```python
from build123d import *

# Parameters (mm, degrees)
SKETCH1_W           = 60
SKETCH1_H           = 50
BOSS_EXTRUDE1_DEPTH = 30
CUT_EXTRUDE1_DEPTH  = 30
BOSS_EXTRUDE2_DEPTH = 20
BOSS_EXTRUDE3_DEPTH = 30


with BuildPart() as part:
    # Sketch1 → Boss-Extrude1 (new body)
    with BuildSketch(Plane(origin=(0, 0, 0), x_dir=(1, 0, 0), z_dir=(0, 1, 0))):
        with Locations((30, 25)):
            Rectangle(SKETCH1_W, SKETCH1_H)
    extrude(amount=BOSS_EXTRUDE1_DEPTH)

    # Sketch2 → Cut-Extrude1 (cut)
    with BuildSketch(Plane(origin=(0, 30, 0), x_dir=(1, 0, 0), z_dir=(0, 1, 0))):
        Polygon((0, 20), (20, 0), (0, 0), align=None)
    extrude(amount=-CUT_EXTRUDE1_DEPTH, mode=Mode.SUBTRACT)

    # Sketch3 → Boss-Extrude2 (add)
    with BuildSketch(Plane(origin=(0, 30, 0), x_dir=(1, 0, 0), z_dir=(0, 1, 0))):
        Polygon((10, 50), (60, 50), (60, 10), (40, 10), (10, 40), align=None)
    extrude(amount=BOSS_EXTRUDE2_DEPTH)

    # Sketch4 → Boss-Extrude3 (add)
    with BuildSketch(Plane(origin=(0, 0, -50), x_dir=(-1, 0, 0), z_dir=(0, 0, -1))):
        Polygon((20, 0), (20, 10), (0, 30), (0, 0), align=None)
    extrude(amount=-BOSS_EXTRUDE3_DEPTH)


solid = part.part
```
Source: CAD feature listing. Evaluate the final solid. Frame: model axes, mm. A direction names the side the tool comes from. Give positions to 0.01 mm unless a question says otherwise; leave off trailing zeros. Loops run counter-clockwise (first coordinate to the right, second up) from the corner with the lowest first, then second, coordinate; pieces in that order, holes last. Notation, with made-up numbers: (67, 52.5) -> (120, 52.5) arc R19 cw to (120, 69.5) -> close; hole circle Ø1 at (9, 7). An arc over 180 degrees is marked (long way). Put each result on its own line as item: value. Start each with the question number.
1) Cut plane B-B (y = 14.5). Return loops of the section in (x, z), then the cut area to 4 significant figures.
2) Cut plane A-A (z = -34). Return loops of the section in (x, y).
3) Reachability of faces 1 (the face through (50, 40, -10)), 2 (the face through (25, 40, -25)), 3 (the face through (10, 40, -45)) from +Z, -Z, +X, -X, +Y, -Y: full face, straight path, thin tool, end or side. Return the list, or none.
4) Cut plane D-D (z = -45). Return loops of the section in (x, y), then the cut area to 3 significant figures.
5) Material intervals for probe 1 along Y at (x, z) = (15, -33.5); probe 2 along X at (y, z) = (20, -36); probe 3 along X at (y, z) = (23, -11.5), sorted ascending.
6) Cut plane C-C (x = 22.5). Return loops of the section in (y, z), then the cut area to 3 significant figures.
7) Contact query for flat-ended pins moving along their axis: P1, Ø3, axis at y = 43.5, z = -30.5, coming from the -X side; P2, Ø11, axis at y = 40, z = -43, coming from the -X side; P3, Ø22, axis at x = -13.5, y = 15, coming from the +Z side. Output: stop coordinate, or through.
Results are:
1. outline: (-15.5, -50) -> (60, -50) -> (60, 0) -> (20, 0) -> (0, -20) -> (-15.5, -20) -> close
1. area: 3,265 mm2
2. outline: (-20, 0) -> (60, 0) -> (60, 50) -> (16, 50) -> (16, 30) -> (0, 30) -> (-20, 10) -> close
3. face 1: +Z, +X, -X, +Y
3. face 2: +Z, -X, +Y
3. face 3: +Z, -Z, -X, +Y
4. outline: (-20, 0) -> (60, 0) -> (60, 50) -> (10, 50) -> (10, 30) -> (0, 30) -> (-20, 10) -> close
4. area: 3,200 mm2
5. probe 1: y = 0 to 30
5. probe 2: x = -10 to 60
5. probe 3: x = 8.5 to 60
6. outline: (0, -50) -> (50, -50) -> (50, -27.5) -> (30, -27.5) -> (30, 0) -> (0, 0) -> close
6. area: 1,950 mm2
7. P1: stops at x = 18
7. P2: stops at x = 10
7. P3: stops at z = -20
